Drawing for the job (mm, zero at the part's lowest x, y, z). Round coordinates to 2 decimals unless told otherwise and drop trailing zeros. Write each loop counter-clockwise with the first axis right and the second up, starting at its lowest first coordinate (ties: lowest second). Pieces come first, ordered by that corner, then holes. Notation, with made-up numbers: M 64.5,37.25 L 113.5,37.25 A31 cw 113.5,68.25 Z; hole C -22.75,38.25 d5. An arc over 180 degrees is marked long. Use a Markdown table: item, result. Add a question column.
1) Wall check: probe 1 along Y at (x, z) = (60, 24.5); probe 2 along X at (y, z) = (1050, 19); probe 3 along Y at (x, z) = (80, 31.5). Give the ranges that are in metal, low to high.
2) Drop flat-ended pins along their axis: P1, Ø3, axis at y = 462, z = 6, coming from the +X side; P2, Ø1, axis at y = 789.5, z = 23.5, coming from the +X side; P3, Ø2, axis at y = 1118.5, z = 29, coming from the +X side. Give the stop position or say it passes through.
3) Slice it at A-A on x = 60. Write the cut outline in (y, z), plus the area to 3 significant figures.
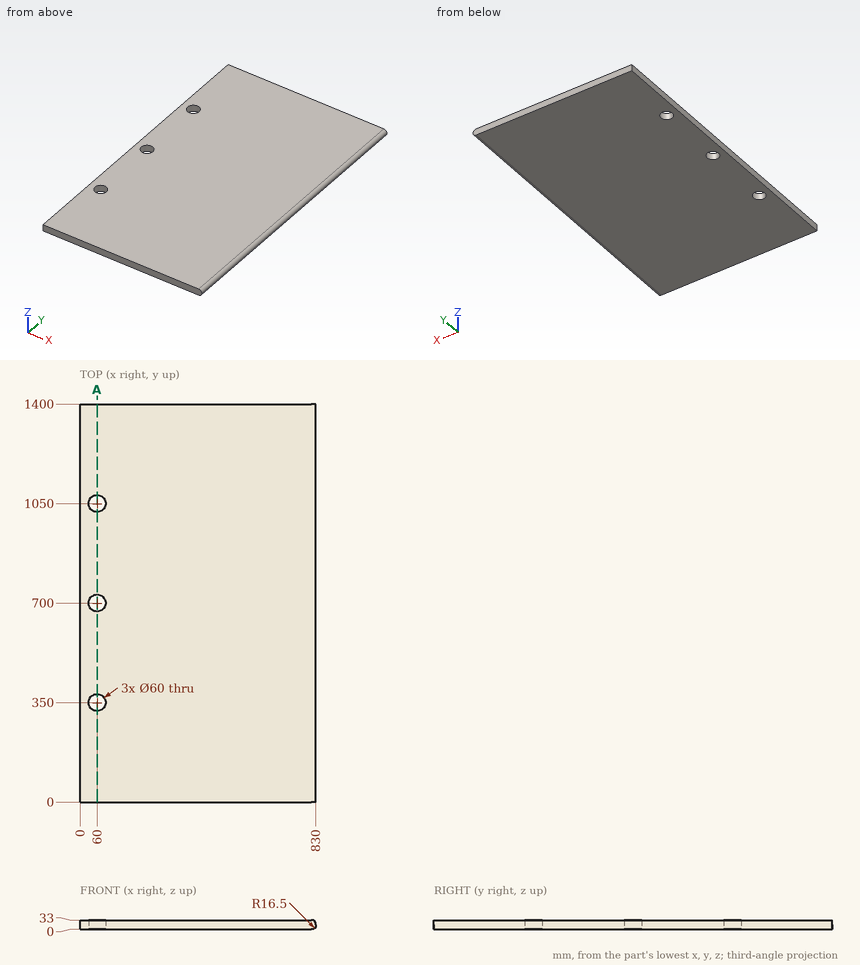
Entries:
| question | item | result |
|---|---|---|
| 1 | probe 1 | y = 0 to 320, 380 to 670, 730 to 1020, 1080 to 1400 |
| 1 | probe 2 | x = 0 to 30, 90 to 829.81 |
| 1 | probe 3 | y = 0 to 327.64, 372.36 to 677.64, 722.36 to 1027.64, 1072.36 to 1400 |
| 2 | P1 | stops at x = 827.33 |
| 2 | P2 | stops at x = 828.67 |
| 2 | P3 | stops at x = 825.33 |
| 3 | outline | M 0,0 L 320,0 L 320,33 L 0,33 Z; M 380,0 L 670,0 L 670,33 L 380,33 Z; M 730,0 L 1020,0 L 1020,33 L 730,33 Z; M 1080,0 L 1400,0 L 1400,33 L 1080,33 Z |
| 3 | area | 40,300 mm^2 |
